Source: CAD feature listing. Evaluate the final solid. Frame: model axes, mm. Face numbers are marked on the shaded views. Give positions to 0.01 mm unless a question says otherwise; leave off trailing zeros. Write each loop counter-clockwise with the first axis right and the second up, starting at its lowest first coordinate (ties: lowest second). Pieces come first, ordered by that corner, then holes.
Autodesk Inventor part; units mm, degrees
ref_plane "YZ Plane" through (0, 0, 0) normal (1, 0, 0) x (0, 1, 0)
ref_plane "XZ Plane" through (0, 0, 0) normal (0, 1, 0) x (-1, 0, 0)
ref_plane "XY Plane" through (0, 0, 0) normal (0, 0, 1) x (1, 0, 0)
sketch "Sketch1" plane through (0, 0, 0) normal (0, 1, 0) x (-1, 0, 0)
  line L0 (-6.35, -3.175) -> (6.35, -3.175)
  line L1 (6.35, -3.175) -> (6.35, 3.175)
  line L2 (6.35, 3.175) -> (-6.35, 3.175)
  line L3 (-6.35, 3.175) -> (-6.35, -3.175)
  line L4 (-6.35, -3.175) -> (6.35, 3.175) construction
  line L5 (6.35, -3.175) -> (-6.35, 3.175) construction
  point P0 (0, 0)
  dimension "d0" = 12.7
  dimension "d1" = 6.35
extrude "Extrusion1" add sketch "Sketch1" along normal blind 6.35
sketch "Sketch2" plane through (0, 6.35, 0) normal (0, 1, 0) x (1, 0, 0)
  line L0 (0, 0) -> (3.175, 0)
  dimension "d4" = 3.175
hole "Hole1" at (3.175, 6.35, 0) direction (0, -1, 0) diameter 5.1054 end up to surface
properties part number "sheild stop" material "Aluminum 6061"
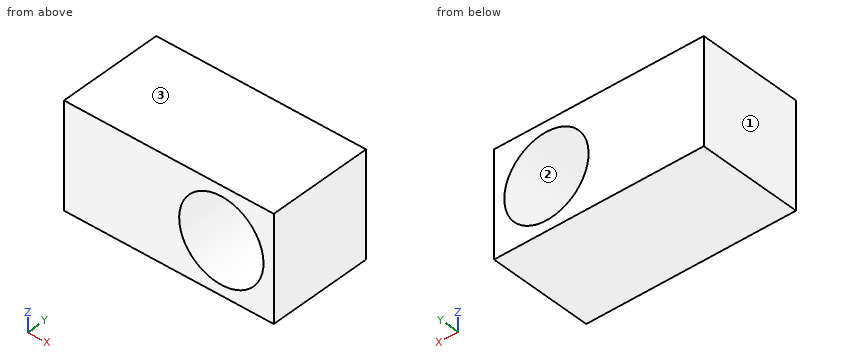
1. Mould query, pull axis Z, two halves, no side actions, for the marked faces 1, 2 and 3. Classes: +Z half, -Z half, draft (parallel to the pull), parting line (faces both ways), or undercut.
2. Cut plane C-C, the plane x = 1.5. Return the cut outline in (y, z) (3 decimals), then the cut area to 3 significant figures.
3. Line query: L1, parallel to X at y = 1.5, z = 0; L2, parallel to Z at x = 3.25, y = 2 (3 decimals); L3, parallel to X at y = 1.75, z = 2.25. Output: solid intervals per line, ascending.
4. Cut plane A-A, the plane z = 0. Return the cut outline in (x, y).
5. Cut plane B-B, the plane y = 2.25. Return the cut outline in (x, z) (3 decimals), then the cut area to 3 significant figures.
Response values:
1. face 1: draft
1. face 2: undercut
1. face 3: +Z half
2. outline: (0, -3.175) - (6.35, -3.175) - (6.35, -1.926) - (0, -1.926) - close; (0, 1.926) - (6.35, 1.926) - (6.35, 3.175) - (0, 3.175) - close
2. area: 15.9 mm2
3. L1: x = -6.35 to 0.62, 5.73 to 6.35
3. L2: z = -3.175 to -2.552, 2.552 to 3.175
3. L3: x = -6.35 to 1.97, 4.38 to 6.35
4. outline: (-6.35, 0) - (0.62, 0) - (0.62, 6.35) - (-6.35, 6.35) - close; (5.73, 0) - (6.35, 0) - (6.35, 6.35) - (5.73, 6.35) - close
5. outline: (-6.35, -3.175) - (6.35, -3.175) - (6.35, 3.175) - (-6.35, 3.175) - close; hole circle Ø5.105 at (3.175, 0)
5. area: 60.2 mm2
